Could you check a few things on this model? Use its own coordinates, in mm. Face numbers are marked on the shaded views. A direction names the side the tool comes from. Round coordinates to 2 decimals unless told otherwise and drop trailing zeros. Write each loop counter-clockwise with the first axis right and the second up, starting at its lowest first coordinate (ties: lowest second). Pieces come first, ordered by that corner, then holes. Notation, with made-up numbers: M 24.25,-15 L 28.25,-15 A10 ccw 28.25,-4 Z; hole C 87,34.5 d10. An arc over 180 degrees is marked long. One line per item, written item: value. Start each with the question number.
(1) I'm going to push flat-ended pins straight in: pin 1 Ø1 at (y, z) = (10, -3) entering from -X; pin 2 Ø5 at (x, z) = (6.5, 2) entering from -Y. Where does each tip first touch, or does it pass through?
(2) I want a section at C-C on z = 2.25. Please give me the cut outline in (x, y).
(3) Which directions (+Z, -Z, +X, -X, +Y, -Y) give clear straight access to the entire face, cutting with the end or side of a thin tool? Please do the marked faces 1 and 2.
(4) If I drill on L1, parallel to Y at x = 0, z = 4.3; L2, parallel to Y at x = 0, z = 2; L3, parallel to Z at x = 1, y = 13, over which ranges is the centre line in solid material (lowest first)?
(5) Thinking about a two-plate mould opening in Y: for the marked faces 3, 4 and 5, which applies, released by +Y, released by -Y, zero draft, split by the parting line, or undercut?
(6) I want a section at D-D on y = 11. Please give me the cut outline in (x, z), and give its area (3 significant figures).
(7) I want a section at A-A on y = 0. Please give me the cut outline in (x, z), and give its area (3 significant figures).
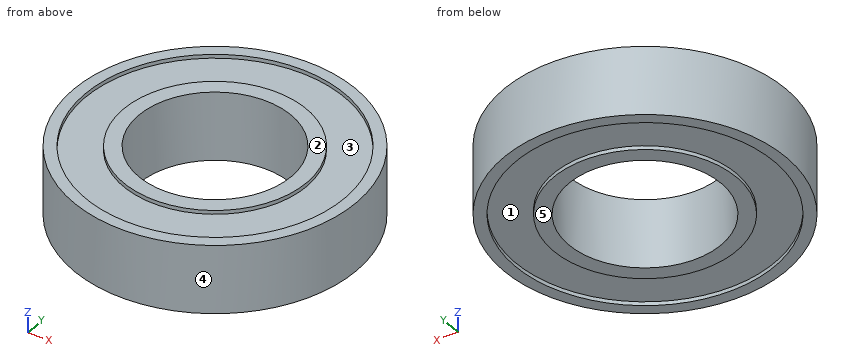
```python
from build123d import *

# Parameters (mm, degrees)
SKETCH_1_R          = 18.5
EXTRUDE_1_DEPTH     = 4.5
SKETCH_2_R          = 10
CUT_EXTRUDE_1_DEPTH = 10
SKETCH_3_R          = 17
SKETCH_3_R_2        = 12
CUT_EXTRUDE_2_DEPTH = 0.5


with BuildPart() as part:
    # 草圖1 → 填料-伸長1 (new body, symmetric)
    with BuildSketch(Plane.XY):
        Circle(SKETCH_1_R)
    extrude(amount=EXTRUDE_1_DEPTH, both=True)

    # 草圖2 → 除料-伸長1 (cut, through all)
    with BuildSketch(Plane.XY.offset(4.5)):
        Circle(SKETCH_2_R)
    extrude(amount=-CUT_EXTRUDE_1_DEPTH, mode=Mode.SUBTRACT)

    # 草圖3 → 除料-伸長2 (cut)
    with BuildSketch(Plane.XY.offset(4.5)):
        Circle(SKETCH_3_R)
        Circle(SKETCH_3_R_2, mode=Mode.SUBTRACT)
    cut_extrude_2 = extrude(amount=-CUT_EXTRUDE_2_DEPTH, mode=Mode.SUBTRACT)

    # 鏡射1: 除料-伸長2 across plane
    add(cut_extrude_2.mirror(Plane.XY), mode=Mode.SUBTRACT)


solid = part.part
```
Found:
1. pin 1: stops at x = -15.87
1. pin 2: stops at y = -18.06
2. outline: C 0,0 d37; hole C 0,0 d20
3. face 1: -Z
3. face 2: +Z, +X, -X, +Y, -Y
4. L1: y = -18.5 to -17, -12 to -10, 10 to 12, 17 to 18.5
4. L2: y = -18.5 to -10, 10 to 18.5
4. L3: z = -4 to 4
5. face 3: undercut
5. face 4: split by the parting line
5. face 5: zero draft
6. outline: M -14.87,-4.5 L -12.96,-4.5 L -12.96,-4 L -4.8,-4 L -4.8,-4.5 L 4.8,-4.5 L 4.8,-4 L 12.96,-4 L 12.96,-4.5 L 14.87,-4.5 L 14.87,4.5 L 12.96,4.5 L 12.96,4 L 4.8,4 L 4.8,4.5 L -4.8,4.5 L -4.8,4 L -12.96,4 L -12.96,4.5 L -14.87,4.5 Z
6. area: 251 mm²
7. outline: M -18.5,-4.5 L -17,-4.5 L -17,-4 L -12,-4 L -12,-4.5 L -10,-4.5 L -10,4.5 L -12,4.5 L -12,4 L -17,4 L -17,4.5 L -18.5,4.5 Z; M 10,-4.5 L 12,-4.5 L 12,-4 L 17,-4 L 17,-4.5 L 18.5,-4.5 L 18.5,4.5 L 17,4.5 L 17,4 L 12,4 L 12,4.5 L 10,4.5 Z
7. area: 143 mm²
